```python
from build123d import *

# Parameters (mm, degrees)
BOSS_EXTRUDE1_DEPTH      = 5
BOSS_EXTRUDE3_DEPTH      = 50
BOSS_EXTRUDE3_DEPTH_BACK = 22
BOSS_EXTRUDE4_DEPTH      = 50
BOSS_EXTRUDE4_DEPTH_BACK = 22
CUT_EXTRUDE3_DEPTH       = 50
SKETCH6_R                = 3.5
CUT_EXTRUDE7_DEPTH       = 74
SKETCH7_R                = 8
CUT_EXTRUDE8_DEPTH       = 35
CUT_EXTRUDE9_DEPTH       = 35


with BuildPart() as part:
    # Sketch1 → Boss-Extrude1 (new body)
    with BuildSketch(Plane(origin=(0, 0, 0), x_dir=(1, 0, 0), z_dir=(0, 1, 0))):
        with BuildLine():
            Line((32.5, 71.691135645), (32.5, 68.476103961))
            ThreePointArc((32.5, 68.476103961), (0, 35.976103961), (-32.5, 68.476103961))
            Line((-32.5, 68.476103961), (-32.5, 71.691135645))
            ThreePointArc((-32.5, 71.691135645), (0, 104.191135645), (32.5, 71.691135645))
        make_face()
        with BuildLine():
            Line((2.75, 98.791135645), (2.75, 96.891135645))
            ThreePointArc((2.75, 96.891135645), (0, 94.141135645), (-2.75, 96.891135645))
            Line((-2.75, 96.891135645), (-2.75, 98.791135645))
            ThreePointArc((-2.75, 98.791135645), (0, 101.541135645), (2.75, 98.791135645))
        make_face(mode=Mode.SUBTRACT)
        with BuildLine():
            Line((20.25, 71.691135645), (20.25, 68.476103961))
            ThreePointArc((20.25, 68.476103961), (0, 48.226103961), (-20.25, 68.476103961))
            Line((-20.25, 68.476103961), (-20.25, 71.691135645))
            ThreePointArc((-20.25, 71.691135645), (0, 91.941135645), (20.25, 71.691135645))
        make_face(mode=Mode.SUBTRACT)
        with BuildLine():
            Line((2.75, 41.376103961), (2.75, 43.276103961))
            ThreePointArc((2.75, 43.276103961), (0, 46.026103961), (-2.75, 43.276103961))
            Line((-2.75, 43.276103961), (-2.75, 41.376103961))
            ThreePointArc((-2.75, 41.376103961), (0, 38.626103961), (2.75, 41.376103961))
        make_face(mode=Mode.SUBTRACT)
        with BuildLine():
            Line((28.355451649, 71.021360387), (28.346988019, 69.121379238))
            ThreePointArc((28.346988019, 69.121379238), (25.584765313, 66.383656513), (22.847042588, 69.145879219))
            Line((22.847042588, 69.145879219), (22.855506218, 71.045860368))
            ThreePointArc((22.855506218, 71.045860368), (25.617728924, 73.783583093), (28.355451649, 71.021360387))
        make_face(mode=Mode.SUBTRACT)
        with BuildLine():
            Line((-28.355451649, 71.021360387), (-28.346988019, 69.121379238))
            ThreePointArc((-28.346988019, 69.121379238), (-25.584765313, 66.383656513), (-22.847042588, 69.145879219))
            Line((-22.847042588, 69.145879219), (-22.855506218, 71.045860368))
            ThreePointArc((-22.855506218, 71.045860368), (-25.617728924, 73.783583093), (-28.355451649, 71.021360387))
        make_face(mode=Mode.SUBTRACT)
    extrude(amount=BOSS_EXTRUDE1_DEPTH)

    # Sketch1_4 → Boss-Extrude3 (add, two sides)
    with BuildSketch(Plane(origin=(0, 0, 0), x_dir=(1, 0, 0), z_dir=(0, 1, 0))) as boss_extrude3_sk:
        with BuildLine():
            Line((34.993484539, 71.691135645), (34.993484539, 68.476103961))
            ThreePointArc((34.993484539, 68.476103961), (0, 33.482619422), (-34.993484539, 68.476103961))
            Line((-34.993484539, 68.476103961), (-34.993484539, 71.691135645))
            ThreePointArc((-34.993484539, 71.691135645), (0, 106.684620184), (34.993484539, 71.691135645))
        make_face()
        with BuildLine():
            Line((32.5, 71.691135645), (32.5, 68.476103961))
            ThreePointArc((32.5, 68.476103961), (0, 35.976103961), (-32.5, 68.476103961))
            Line((-32.5, 68.476103961), (-32.5, 71.691135645))
            ThreePointArc((-32.5, 71.691135645), (0, 104.191135645), (32.5, 71.691135645))
        make_face(mode=Mode.SUBTRACT)
    extrude(amount=BOSS_EXTRUDE3_DEPTH)
    extrude(boss_extrude3_sk.sketch, amount=-BOSS_EXTRUDE3_DEPTH_BACK)

    # Sketch2 → Boss-Extrude4 (add, two sides)
    with BuildSketch(Plane(origin=(0, 0, 0), x_dir=(1, 0, 0), z_dir=(0, 1, 0))) as boss_extrude4_sk:
        with BuildLine():
            Line((-15.85, 22.838532478), (-14.442663196, 22.838532478))
            Line((-14.442663196, 22.838532478), (-14.977598698, 15.918189547))
            Line((-14.977598698, 15.918189547), (-25.022401302, 15.918189547))
            Line((-25.022401302, 15.918189547), (-25.557336804, 22.838532478))
            Line((-25.557336804, 22.838532478), (-24.15, 22.838532478))
            Line((-24.15, 22.838532478), (-24.15, 27.083619803))
            Line((-24.15, 27.083619803), (-25.25, 27.083619803))
            Line((-25.25, 27.083619803), (-39, 27.083619803))
            Line((-39, 27.083619803), (-34.964708316, 70.119775602))
            ThreePointArc((-34.964708316, 70.119775602), (0, 36.691135645), (34.964708316, 70.119775602))
            Line((34.964708316, 70.119775602), (39, 27.083619803))
            Line((39, 27.083619803), (25.25, 27.083619803))
            Line((25.25, 27.083619803), (24.15, 27.083619803))
            Line((24.15, 27.083619803), (24.15, 22.838532478))
            Line((24.15, 22.838532478), (25.557336804, 22.838532478))
            Line((25.557336804, 22.838532478), (25.022401302, 15.918189547))
            Line((25.022401302, 15.918189547), (14.977598698, 15.918189547))
            Line((14.977598698, 15.918189547), (14.442663196, 22.838532478))
            Line((14.442663196, 22.838532478), (15.85, 22.838532478))
            Line((15.85, 22.838532478), (15.85, 27.083619803))
            Line((15.85, 27.083619803), (14.75, 27.083619803))
            Line((14.75, 27.083619803), (-14.75, 27.083619803))
            Line((-14.75, 27.083619803), (-15.85, 27.083619803))
            Line((-15.85, 27.083619803), (-15.85, 22.838532478))
        make_face()
    extrude(amount=BOSS_EXTRUDE4_DEPTH)
    extrude(boss_extrude4_sk.sketch, amount=-BOSS_EXTRUDE4_DEPTH_BACK)

    # Sketch8 → Cut-Extrude3 (cut, symmetric)
    with BuildSketch(Plane(origin=(0, 0, 0), x_dir=(0, 0, -1), z_dir=(1, 0, 0))):
        Polygon((15.918189547, 50), (106.684620184, 50), (106.684620184, 16.610675261), align=None)
        with BuildLine():
            Line((106.684620184, 0), (106.684620184, -22))
            Line((106.684620184, -22), (40.588201897, -22))
            add(Edge.make_bspline(
                [(106.684620184, 0), (69.600838441, -0.610728102), (40.588201897, -22)],
                knots=[0, 0, 0, 1, 1, 1], degree=2))
        make_face()
    extrude(amount=CUT_EXTRUDE3_DEPTH, both=True, mode=Mode.SUBTRACT)

    # Sketch6 → Cut-Extrude7 (cut)
    with BuildSketch(Plane.XY.offset(-70)):
        with Locations((-20, -10.130588175)):
            Circle(SKETCH6_R)
        with Locations((20, -10.130588175)):
            Circle(SKETCH6_R)
    extrude(amount=CUT_EXTRUDE7_DEPTH, mode=Mode.SUBTRACT)

    # Sketch7 → Cut-Extrude8 (cut)
    with BuildSketch(Plane.XY.offset(-70)):
        with Locations((-20, -10.125507159)):
            Circle(SKETCH7_R)
        with Locations((20, -10.125507159)):
            Circle(SKETCH7_R)
    extrude(amount=CUT_EXTRUDE8_DEPTH, mode=Mode.SUBTRACT)

    # Sketch4 → Cut-Extrude9 (cut)
    with BuildSketch(Plane(origin=(0, 0, 0), x_dir=(1, 0, 0), z_dir=(0, 1, 0))):
        Polygon((25.88119751, 27.083619803), (-2e-09, 27.101118051), (-25.88119751, 27.083619803), (-32.125, 22.89108437), (-32.33386562, 13.718189547), (0, 13.918189547), (32.33386562, 13.718189547), (32.125, 22.89108437), align=None)
    extrude(amount=-CUT_EXTRUDE9_DEPTH, mode=Mode.SUBTRACT)


solid = part.part
```
Here's how the part is built. I have some questions about the finished solid (model axes, mm). A direction names the side the tool comes from. Round coordinates to 2 decimals unless told otherwise and drop trailing zeros. Loops run counter-clockwise (first coordinate to the right, second up) from the corner with the lowest first, then second, coordinate; pieces in that order, holes last.
1. Will these pins go through, and if not, where does the flat tip stop? pin 1 (3.5 mm diameter, centred on y = -4.5, z = -70.5, fed in from +X); pin 2 (3 mm diameter, centred on x = -13.5, y = -14, fed in from -Z); pin 3 (1.5 mm diameter, centred on x = -15, y = 15.5, fed in from -Z).
Answers:
pin 1: stops at x = 35.09
pin 2: stops at z = -39.61
pin 3: stops at z = -103.65
2. If I drill on probe 1 along X at (y, z) = (4, -70.5); probe 2 along Y at (x, z) = (-12, -41); probe 3 along X at (y, z) = (-8, -62.5), over which ranges is the centre line in solid material (lowest first)?
Answers:
probe 1: x = -34.99 to -28.35, -22.85 to -20.25, 20.25 to 22.85, 28.35 to 34.99
probe 2: y = 0 to 5
probe 3: x = -35.68 to -31.95, 31.95 to 35.68
3. Suppose I cut it at A-A, the plane y = 9.5. Please give me the cut outline in (x, z), and give its area (3 significant figures).
Answers:
outline: (-39, -27.08) - (-34.99, -69.81) - (-34.99, -71.69) arc R34.99 ccw to (34.99, -71.69) - (34.99, -69.81) - (39, -27.08) - (24.15, -27.08) - (24.15, -22.84) - (25.56, -22.84) - (25.02, -15.92) - (14.98, -15.92) - (14.44, -22.84) - (15.85, -22.84) - (15.85, -27.08) - (-15.85, -27.08) - (-15.85, -22.84) - (-14.44, -22.84) - (-14.98, -15.92) - (-25.02, -15.92) - (-25.56, -22.84) - (-24.15, -22.84) - (-24.15, -27.08) - close; hole (-32.5, -71.69) arc R32.5 ccw to (32.5, -71.69) - (32.5, -68.48) arc R32.5 ccw to (21.2, -43.84) arc R35 ccw to (-21.2, -43.84) arc R32.5 ccw to (-32.5, -68.48) - close
area: 1,930 mm2
4. Thinking about a two-plate mould opening in Y: for faces 1 (the face through (-0.06, 2.46, -101.54)), 2 (the face through (-18.12, -7.18, -31.1)), 3 (the face through (-0.18, 43.12, -34.62)), which applies, released by +Y, released by -Y, zero draft, split by the parting line, or undercut?
Answers:
face 1: zero draft
face 2: undercut
face 3: released by +Y
5. For faces 4 (the face through (-18, -14, -35)), 5 (the face through (-20.25, 2, -70)), 6 (the face through (32.5, -3, -70)), 7 (the face through (-32.5, 18, -70)), which set-ups out of +Z, -Z, +X, -X, +Y, -Y let a thin tool reach every point of the face, with its end or its side?
Answers:
face 4: -Z
face 5: +Y, -Y
face 6: -Y
face 7: +Y
